Here's the drawing with two shaded views (mm, measured from the low corner). I have some questions. A direction names the side the tool comes from. Round coordinates to 2 decimals unless told otherwise and drop trailing zeros. Write each loop counter-clockwise with the first axis right and the second up, starting at its lowest first coordinate (ties: lowest second). Pieces come first, ordered by that corner, then holes. Notation, with made-up numbers: M 72,14 L 102,14 A23 ccw 102,31 Z; hole C -17,63.25 d6. An arc over 180 degrees is marked long. Write item = value, one per line. Start each with the question number.
(1) I need wall thicknesses on line 1 along Y through (x, z) = (3.5, 0.5); line 2 along Z through (x, y) = (4.25, 8); line 3 along X through (y, z) = (14, 3.5). Which ranges of each line are inside material? Lowest first, please.
(2) Will these pins go through, and if not, where does the flat tip stop? pin 1 Ø1.5 at (y, z) = (67, 6.5) entering from -X; pin 2 Ø1 at (x, y) = (6, 35) entering from -Z; pin 3 Ø1.5 at (x, y) = (6.5, 9) entering from -Z.
(3) I want a section at A-A (z = 3.95). List the corners of the cut face in (x, y) for me (3 decimals), and give its area (3 significant figures).
(4) I want a section at B-B (x = 3.95). List the corners of the cut face in (y, z) for me (3 decimals), and give its area (3 significant figures).
(5) On a 3-axis mill with a long thin cutter (end or side, diameter ignored), from which of +Z, -Z, +X, -X, +Y, -Y can I reach the whole of each face in a straight line? I mean the marked faces 1, 2 and 3. Say none if no direction works.
(6) I want a section at C-C (y = 75). List the corners of the cut face in (x, z) for me.
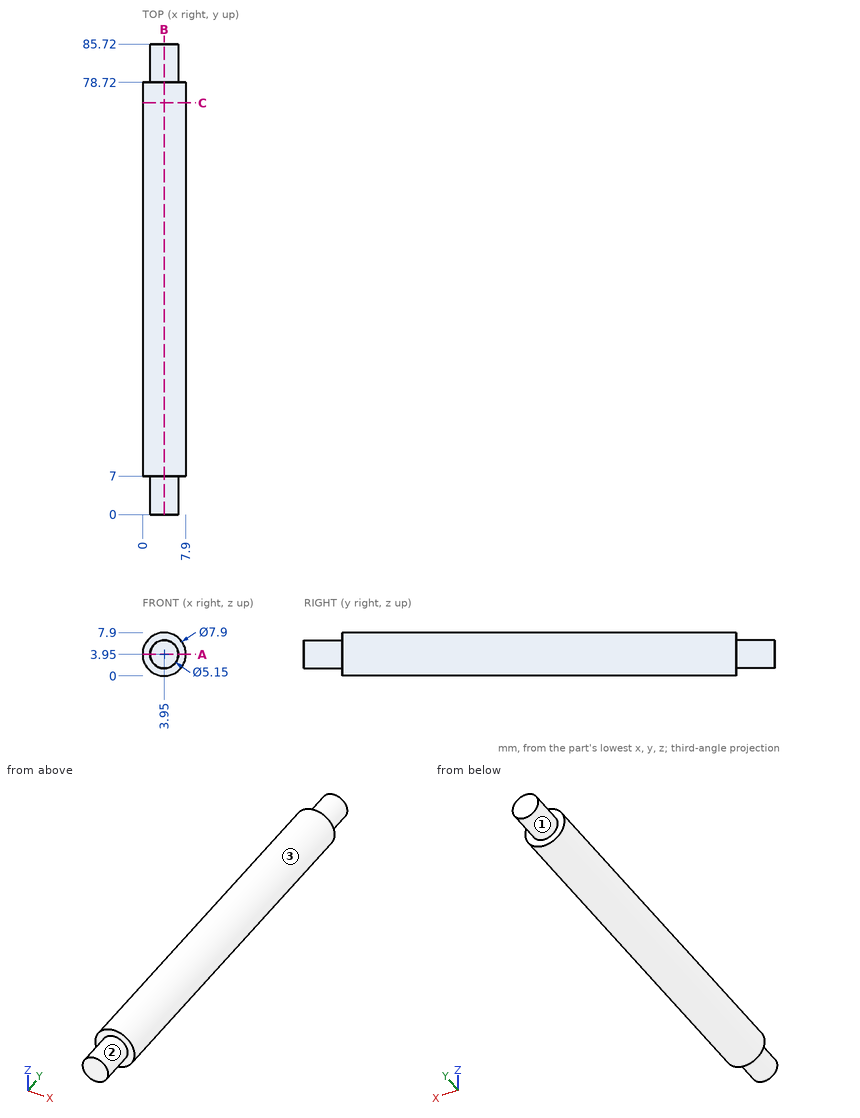
Returned:
q1.line_1 = 7 to 78.72
q1.line_2 = 0.01 to 7.89
q1.line_3 = 0.03 to 7.87
q2.pin_1 = 0.43
q2.pin_2 = 0.32
q2.pin_3 = 0.43
q3.outline = M 0,7 L 1.375,7 L 1.375,0 L 6.525,0 L 6.525,7 L 7.9,7 L 7.9,78.72 L 6.525,78.72 L 6.525,85.72 L 1.375,85.72 L 1.375,78.72 L 0,78.72 Z
q3.area = 639 mm²
q4.outline = M 0,1.375 L 7,1.375 L 7,0 L 78.72,0 L 78.72,1.375 L 85.72,1.375 L 85.72,6.525 L 78.72,6.525 L 78.72,7.9 L 7,7.9 L 7,6.525 L 0,6.525 Z
q4.area = 639 mm²
q5.face_1 = +Y
q5.face_2 = -Y
q5.face_3 = +Y, -Y
q6.outline = C 3.95,3.95 d7.9
